Here's how the part is built. I have some questions about the finished solid (model axes, mm). A direction names the side the tool comes from. Round coordinates to 2 decimals unless told otherwise and drop trailing zeros. Write each loop counter-clockwise with the first axis right and the second up, starting at its lowest first coordinate (ties: lowest second). Pieces come first, ordered by that corner, then holes. Notation, with made-up numbers: M 63.5,78.5 L 115.5,78.5 A20 cw 115.5,106.5 Z; hole C 6.25,11.5 d11. An arc over 180 degrees is marked long. Write item = value, one per line. Start each with the question number.
(1) Will these pins go through, and if not, where does the flat tip stop? pin 1 Ø5 at (y, z) = (-51, 16) entering from +X; pin 2 Ø8 at (x, z) = (25.5, 5) entering from -Y; pin 3 Ø3 at (x, z) = (-1, 2.5) entering from +Y.
(2) I want a section at C-C (z = 8.75). List the corners of the cut face in (x, y) for me.
(3) I want a section at B-B (y = -46). List the corners of the cut face in (x, z) for me, and give its area (3 significant figures).
(4) On a 3-axis mill with a long thin cutter (end or side, diameter ignored), from which of +Z, -Z, +X, -X, +Y, -Y can I reach the whole of each face in a straight line? I mean faces 5 (the flat face through (15, 24.286, 2)), 6 (the flat face through (14, -57.514, 2)), 7 (the flat face through (9, -47.514, 2)), 8 (the flat face through (-25.192, -16, 17)). Say none if no direction works.
(5) I want a section at D-D (x = -23.5). List the corners of the cut face in (y, z) for me.
(6) If we mould it in two halves opening along X, with no side actions, what happens to faces 1 (the flat face through (50.685, -17, 2)), 2 (the flat face through (-23, 18.363, 17)), 3 (the flat face through (9, 14.286, 2)), 4 (the flat face through (40.685, -17, 2))? For each: released by +X, released by -X, zero draft, split by the parting line, or undercut.
(7) I want a section at A-A (x = 20.5). List the corners of the cut face in (y, z) for me, and give its area (3 significant figures).
(8) I need wall thicknesses on line 1 along X through (y, z) = (-29, 2.75); line 2 along X through (y, z) = (-26, 6.75); line 3 along X through (y, z) = (36, 10). Which ranges of each line are inside material? Lowest first, please.
```python
from build123d import *

# Parameters (mm, degrees)
F1_W      = 61.8
F1_H      = 61.8
F1_W_2    = 10
F1_H_2    = 46.907837
F2_DEPTH  = 4
F3_W      = 10
F3_H      = 48.056386
F4_DEPTH  = 25
F4_FACE_W = 10
F4_FACE_H = 29
F5_DEPTH  = 157.4
F6_W      = 4.076856
F6_H      = 61.8
F6_H_2    = 4.076856
F7_DEPTH  = 25


with BuildPart() as f2:
    # F1 (on Top) → F2 (new body)
    with BuildSketch(Plane.XY):
        Polygon((50.684865, 24.286445), (-31.115135, 24.286445), (-31.115135, -57.513555), (-21.115135, -57.513555), (50.684865, -57.513555), align=None)
        with Locations((9.784865, -16.613555)):
            Rectangle(F1_W, F1_H, mode=Mode.SUBTRACT)
        with Locations((-26.115135, -80.967473)):
            Rectangle(F1_W_2, F1_H_2)
    extrude(amount=F2_DEPTH)

    # F3 (on face) → F4 (join)
    with BuildSketch(Plane.XY.offset(4)):
        with Locations((-26.115135, -80.393199)):
            Rectangle(F3_W, F3_H)
    extrude(amount=F4_DEPTH)

    # F4_face (on face) → F5 (join)
    with BuildSketch(Plane(origin=(-26.115135, -104.421392, 14.5), x_dir=(1, 0, 0), z_dir=(0, -1, 0))):
        Rectangle(F4_FACE_W, F4_FACE_H)
    extrude(amount=-F5_DEPTH)

    # F6 (on face) → F7 (cut)
    with BuildSketch(Plane.XY.offset(29)):
        with Locations((-23.153563, -16.613555)):
            Rectangle(F6_W, F6_H)
        with Locations((-23.153563, 16.324873)):
            Rectangle(F6_W, F6_H_2)
        with Locations((-23.153563, -49.551983)):
            Rectangle(F6_W, F6_H_2)
    extrude(amount=-F7_DEPTH, mode=Mode.SUBTRACT)


solid = f2.part
```
Returned:
q1.pin_1 = -21.12
q1.pin_2 = -57.51
q1.pin_3 = 24.29
q2.outline = M -31.12,-104.42 L -21.12,-104.42 L -21.12,-51.59 L -25.19,-51.59 L -25.19,18.36 L -21.12,18.36 L -21.12,52.98 L -31.12,52.98 Z
q3.outline = M -31.12,0 L -21.12,0 L -21.12,4 L -25.19,4 L -25.19,29 L -31.12,29 Z; M 40.68,0 L 50.68,0 L 50.68,4 L 40.68,4 Z
q3.area = 228 mm²
q4.face_5 = +Z, -Z, +X, +Y
q4.face_6 = +Z, -Z, +X, -Y
q4.face_7 = +Z, -Z
q4.face_8 = +Z, +X
q5.outline = M -104.42,0 L 52.98,0 L 52.98,29 L 18.36,29 L 18.36,4 L -51.59,4 L -51.59,29 L -104.42,29 Z
q6.face_1 = released by +X
q6.face_2 = zero draft
q6.face_3 = undercut
q6.face_4 = undercut
q7.outline = M -57.51,0 L -47.51,0 L -47.51,4 L -57.51,4 Z; M 14.29,0 L 24.29,0 L 24.29,4 L 14.29,4 Z
q7.area = 80.0 mm²
q8.line_1 = -31.12 to -21.12, 40.68 to 50.68
q8.line_2 = -31.12 to -25.19
q8.line_3 = -31.12 to -21.12
